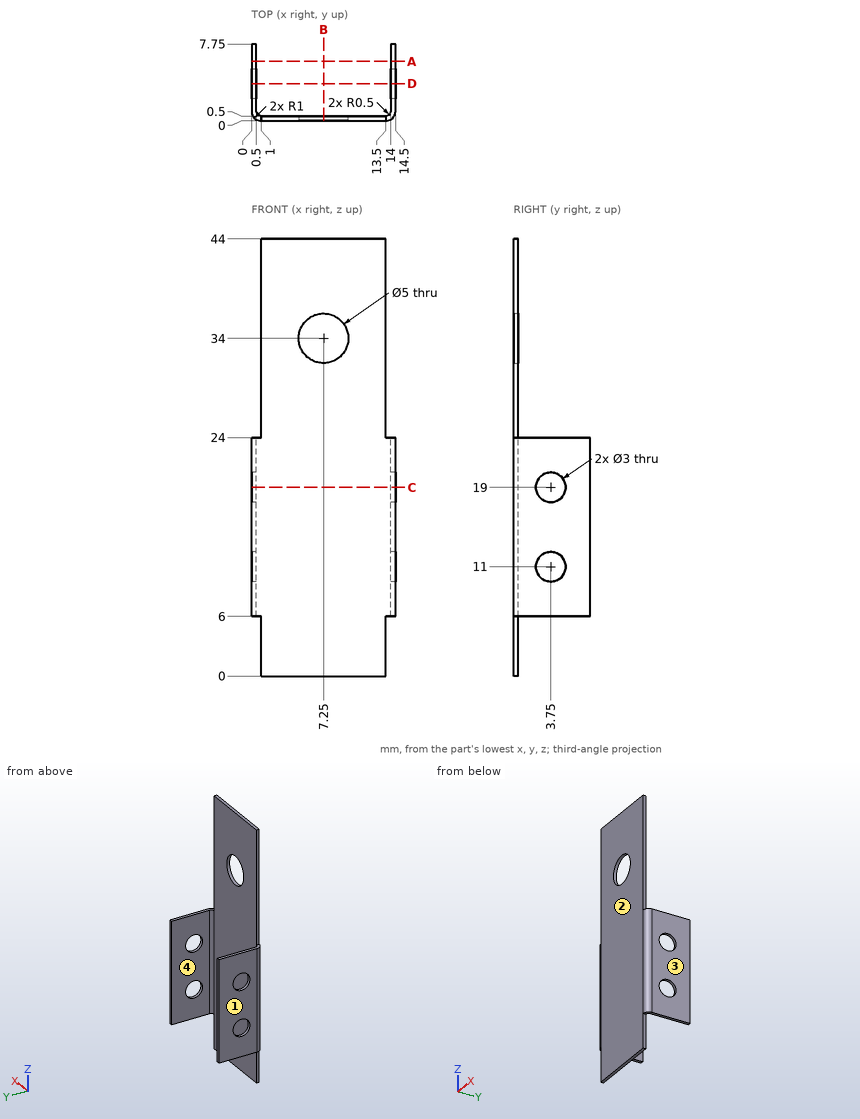
Answer from the drawing. Dimensions are ordinates in mm from the lowest x, y and z of the part. Coordinates: 2 decimals unless noted, no trailing zeros. Order: outer loops, then holes, each group sorted by start corner. A loop starts at its lowest first (then second) coordinate and runs counter-clockwise, first axis right, second up. Notation, with made-up numbers: (41.25, 0) - (64.25, 0) arc R13 cw to (64.25, 22) - close; hole circle Ø5 at (82, 33). An arc over 180 degrees is marked (long way). Put each result on its own line as item: value. Start each with the question number.
1) Find section A-A (y = 6). Give the vertices of the cut face in (x, z).
2) For a pull along X with two mould halves and no side action, classify the marked faces 1, 2, 3 and 4 as released by +X, released by -X, zero draft, split by the parting line, or undercut.
3) Find section C-C (z = 19). Give the vertices of the cut face in (x, y), plus the area to 3 significant figures.
4) Flat-ended cylindrical pins translate along their axes: pin 1 (0.8 mm diameter, centred on x = 14, y = 4, fed in from -Z); pin 2 (0.6 mm diameter, centred on y = 0, z = 39, fed in from +X); pin 3 (0.6 mm diameter, centred on y = 0, z = 2.5, fed in from -X). Find the tip coordinate at first contact, or state that the pin passes through.
5) Find section D-D (y = 3.75). Give the vertices of the cut face in (x, z), plus the area to 3 significant figures.
6) Find the intervals of material crossed by line 1 (Z direction, x = 0.1, y = 3.75); line 2 (X direction, y = 2, z = 13.5); line 3 (Y direction, x = 5.5, z = 6), in increasing order. Write a range as from..to.
7) Find section B-B (x = 7.25). Give the vertices of the cut face in (y, z).
Results list:
1. outline: (0, 6) - (0.5, 6) - (0.5, 24) - (0, 24) - close; (14, 6) - (14.5, 6) - (14.5, 24) - (14, 24) - close
2. face 1: released by -X
2. face 2: zero draft
2. face 3: released by +X
2. face 4: undercut
3. outline: (0, 1) arc R1 ccw to (1, 0) - (13.5, 0) arc R1 ccw to (14.5, 1) - (14.5, 2.25) - (14, 2.25) - (14, 1) arc R0.5 cw to (13.5, 0.5) - (1, 0.5) arc R0.5 cw to (0.5, 1) - (0.5, 2.25) - (0, 2.25) - close; (0, 5.25) - (0.5, 5.25) - (0.5, 7.75) - (0, 7.75) - close; (14, 5.25) - (14.5, 5.25) - (14.5, 7.75) - (14, 7.75) - close
3. area: 11.2 mm^2
4. pin 1: stops at z = 6
4. pin 2: stops at x = 13.5
4. pin 3: stops at x = 1
5. outline: (0, 6) - (0.5, 6) - (0.5, 9.5) - (0, 9.5) - close; (0, 12.5) - (0.5, 12.5) - (0.5, 17.5) - (0, 17.5) - close; (0, 20.5) - (0.5, 20.5) - (0.5, 24) - (0, 24) - close; (14, 6) - (14.5, 6) - (14.5, 9.5) - (14, 9.5) - close; (14, 12.5) - (14.5, 12.5) - (14.5, 17.5) - (14, 17.5) - close; (14, 20.5) - (14.5, 20.5) - (14.5, 24) - (14, 24) - close
5. area: 12.0 mm^2
6. line 1: z = 6..9.5, 12.5..17.5, 20.5..24
6. line 2: x = 0..0.5, 14..14.5
6. line 3: y = 0..0.5
7. outline: (0, 0) - (0.5, 0) - (0.5, 31.5) - (0, 31.5) - close; (0, 36.5) - (0.5, 36.5) - (0.5, 44) - (0, 44) - close
